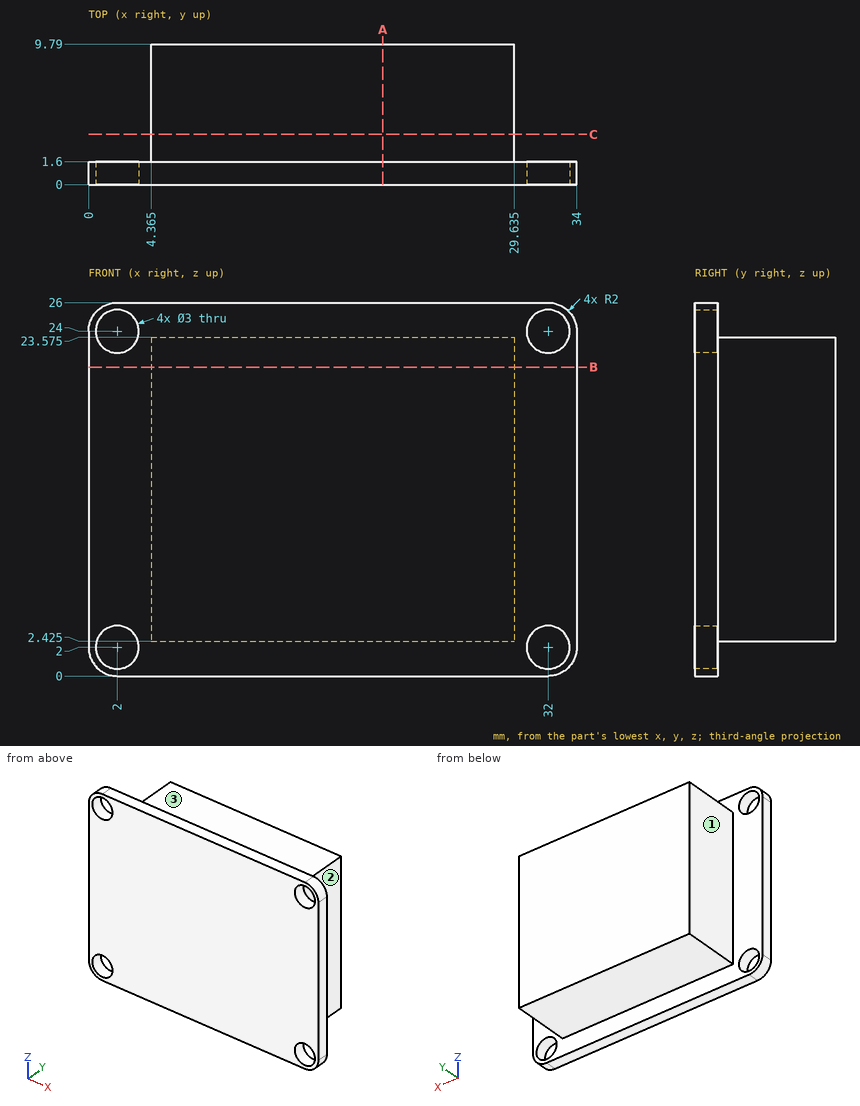
Source: three-view drawing plus pictorial views. Frame: mm from the lowest corner of the part. A direction names the side the tool comes from. Round coordinates to 2 decimals unless told otherwise and drop trailing zeros. Loops run counter-clockwise (first coordinate to the right, second up) from the corner with the lowest first, then second, coordinate; pieces in that order, holes last. Notation, with made-up numbers: (-14, 44.25) - (45, 44.25) arc R19 cw to (45, 59.25) - close; hole circle Ø3 at (72.5, 77). An arc over 180 degrees is marked (long way). Write item = value, one per line. Start each with the question number.
Item 1: Reachability of the marked faces 1, 2 and 3 from +Z, -Z, +X, -X, +Y, -Y: full face, straight path, thin tool, end or side. Return the list, or none.
Item 2: Section query C-C on y = 3.5. Output: boundary loops of the cut face in (x, z) (3 decimals).
Item 3: Section query B-B on z = 21.5. Output: boundary loops of the cut face in (x, y) (3 decimals), plus the area to 3 significant figures.
Item 4: Material intervals for line 1 (Z direction, x = 32, y = 0.95); line 2 (X direction, y = 1.1, z = 24); line 3 (Z direction, x = 24.5, y = 2.75) (3 decimals), sorted ascending.
Item 5: Section query A-A on x = 20.5. Output: boundary loops of the cut face in (y, z) (3 decimals).
Item 6: First-contact query: pin 1 Ø3.5 at (x, z) = (32, 2) entering from +Y; pin 2 Ø1 at (y, z) = (4.5, 21) entering from +X (3 decimals); pin 3 Ø1.5 at (x, y) = (14.5, 3) entering from +Z (3 decimals). Flat tips, straight axial feed; report the tip coordinate or a pass-through.
Results list:
q1.face_1 = +Z, -Z, -X, +Y
q1.face_2 = +Z, -Z, +X, +Y
q1.face_3 = +Z, +X, -X, +Y
q2.outline = (4.365, 2.425) - (29.635, 2.425) - (29.635, 23.575) - (4.365, 23.575) - close
q3.outline = (0, 0) - (34, 0) - (34, 1.6) - (29.635, 1.6) - (29.635, 9.79) - (4.365, 9.79) - (4.365, 1.6) - (0, 1.6) - close
q3.area = 261 mm²
q4.line_1 = 0 to 0.5, 3.5 to 22.5, 25.5 to 26
q4.line_2 = 0 to 0.5, 3.5 to 30.5, 33.5 to 34
q4.line_3 = 2.425 to 23.575
q5.outline = (0, 0) - (1.6, 0) - (1.6, 2.425) - (9.79, 2.425) - (9.79, 23.575) - (1.6, 23.575) - (1.6, 26) - (0, 26) - close
q6.pin_1 = 1.6
q6.pin_2 = 29.635
q6.pin_3 = 23.575
